Check sheet for the modelled part. Datum: model origin and axes. Units: mm. A direction names the side the tool comes from. Round coordinates to 2 decimals unless told otherwise and drop trailing zeros. Write each loop counter-clockwise with the first axis right and the second up, starting at its lowest first coordinate (ties: lowest second). Pieces come first, ordered by that corner, then holes.
Item 1: Set-up check for faces 1 (the flat face through (9, 6, -7.1)), 2 (the cylindrical face through (19.07, 8.35, -1.01)), 3 (the flat face through (24, 13.5, -2)): record each of +Z, -Z, +X, -X, +Y, -Y from which the full face is reachable in a straight line by a thin tool's end or side.
Item 2: Section check D-D, the plane x = 23. Record the cut outline in (y, z), plus the area to 3 significant figures.
Item 3: Section check C-C, the plane y = 20. Record the cut outline in (x, z), plus the area to 3 significant figures.
Item 4: Section check A-A, the plane z = -15.1. Record the cut outline in (x, y), plus the area to 3 significant figures.
Item 5: Material ranges on line 1 along X through (y, z) = (47, -34); line 2 along X through (y, z) = (20, -0.7); line 3 along Y through (x, z) = (6.5, -0.85), recorded low to high.
Item 6: Depth check by flat-ended pin: pin 1 (5.5 mm diameter, centred on x = 8, z = -34.1, fed in from -Y); pin 2 (5.5 mm diameter, centred on x = 8, z = -15.1, fed in from +Y); pin 3 (4 mm diameter, centred on x = 17.5, y = 31, fed in from -Z). Enter the tip coordinate at first touch or a pass-through.
Item 7: Section check B-B, the plane y = 38. Record the cut outline in (x, z).
Item 8: Release check for a two-part mould opening along X. For faces 4 (the flat face through (0, 39, -16)), 5 (the cylindrical face through (26.084, 22.703, -1.014)), 6 (the flat face through (35, 39, -16)), 7 (the flat face through (17, 44, -42.1)) record: pulls with the +X half, pulls with the -X half, needs draft (parallel to the pull), parting line crosses it, or undercut.
from build123d import *

# Parameters (mm, degrees)
BOSS_EXTRUDE1_DEPTH                = 35
MOTOR_START                        = -7.1
MOTOR_MOUNT_BOLT_HOLES_OUTLINE_R   = 1.7
MOTOR_MOUNT_BOLT_HOLES_OUTLINE_R_2 = 9
MOTOR_MOUNT_BOLT_HOLES_DEPTH       = 7.1
MOTOR_COUNTERSINK_DEPTH            = 5.1
MOTOR_COUNTERSINK_DEPTH_BACK       = 2
MOTOR_COUNTERSINK_START            = -7.1
SKETCH2_5_R                        = 15
SKETCH3_R                          = 1.7
CUT_EXTRUDE3_DEPTH                 = 65.980073869


# Read off the part's stored shape, not the designer's step: Motor mount bolt holes
with BuildPart() as part:
    # Sketch1 → Boss-Extrude1 (new body)
    with BuildSketch(Plane(origin=(0, 0, 0), x_dir=(0, 0, -1), z_dir=(1, 0, 0))):
        Polygon((0, 0), (7.1, 0), (7.1, 35), (42.1, 35), (42.1, 53.75), (0, 53.75), align=None)
    extrude(amount=BOSS_EXTRUDE1_DEPTH)

    # Motor mount bolt holes outline → Motor mount bolt holes (cut)
    with BuildSketch(Plane.XY.offset(MOTOR_START)):
        with Locations((17.5, 9)):
            Circle(MOTOR_MOUNT_BOLT_HOLES_OUTLINE_R)
        with Locations((28.5, 20)):
            Circle(MOTOR_MOUNT_BOLT_HOLES_OUTLINE_R)
        with Locations((17.5, 31)):
            Circle(MOTOR_MOUNT_BOLT_HOLES_OUTLINE_R)
        with Locations((17.5, 20)):
            Circle(MOTOR_MOUNT_BOLT_HOLES_OUTLINE_R_2)
        with Locations((6.5, 20)):
            Circle(MOTOR_MOUNT_BOLT_HOLES_OUTLINE_R)
    extrude(amount=MOTOR_MOUNT_BOLT_HOLES_DEPTH, mode=Mode.SUBTRACT)

    # Sketch2<5> → Motor Countersink (cut, two sides: drawn at the far end of the back side and taken through both)
    with BuildSketch(Plane.XY.offset(MOTOR_COUNTERSINK_START - MOTOR_COUNTERSINK_DEPTH_BACK)):
        with Locations((17.5, 20)):
            Circle(SKETCH2_5_R)
    extrude(amount=MOTOR_COUNTERSINK_DEPTH + MOTOR_COUNTERSINK_DEPTH_BACK, mode=Mode.SUBTRACT)

    # Sketch3 → Cut-Extrude3 (cut, through all)
    with BuildSketch(Plane.XZ.offset(-35)):
        with Locations(Location((8, -15.1, 0), (0, 0, 270))):
            Circle(SKETCH3_R)
        with Locations(Location((27, -15.1, 0), (0, 0, 90))):
            Circle(SKETCH3_R)
        with Locations(Location((27, -34.1, 0), (0, 0, 270))):
            Circle(SKETCH3_R)
        with Locations(Location((8, -34.1, 0), (0, 0, 90))):
            Circle(SKETCH3_R)
    extrude(amount=-CUT_EXTRUDE3_DEPTH, mode=Mode.SUBTRACT)


solid = part.part
Values found:
1. face 1: -Z, +X, -X, -Y
1. face 2: +Z, -Z
1. face 3: -Z
2. outline: (0, -7.1) - (6.04, -7.1) - (6.04, -2) - (12.88, -2) - (12.88, 0) - (0, 0) - close; (27.12, -2) - (33.96, -2) - (33.96, -7.1) - (35, -7.1) - (35, -42.1) - (53.75, -42.1) - (53.75, 0) - (27.12, 0) - close
2. area: 867 mm2
3. outline: (0, -7.1) - (2.5, -7.1) - (2.5, -2) - (4.8, -2) - (4.8, 0) - (0, 0) - close; (8.2, -2) - (8.5, -2) - (8.5, 0) - (8.2, 0) - close; (26.5, -2) - (26.8, -2) - (26.8, 0) - (26.5, 0) - close; (30.2, -2) - (32.5, -2) - (32.5, -7.1) - (35, -7.1) - (35, 0) - (30.2, 0) - close
3. area: 45.9 mm2
4. outline: (0, 35) - (6.3, 35) - (6.3, 53.75) - (0, 53.75) - close; (9.7, 35) - (25.3, 35) - (25.3, 53.75) - (9.7, 53.75) - close; (28.7, 35) - (35, 35) - (35, 53.75) - (28.7, 53.75) - close
4. area: 529 mm2
5. line 1: x = 0 to 6.3, 9.7 to 25.3, 28.7 to 35
5. line 2: x = 0 to 4.8, 8.2 to 8.5, 26.5 to 26.8, 30.2 to 35
5. line 3: y = 0 to 18.3, 21.7 to 53.75
6. pin 1: stops at y = 35
6. pin 2: stops at y = 53.75
6. pin 3: stops at z = -2
7. outline: (0, -42.1) - (35, -42.1) - (35, 0) - (0, 0) - close; hole circle Ø3.4 at (8, -34.1); hole circle Ø3.4 at (8, -15.1); hole circle Ø3.4 at (27, -34.1); hole circle Ø3.4 at (27, -15.1)
8. face 4: pulls with the -X half
8. face 5: undercut
8. face 6: pulls with the +X half
8. face 7: needs draft
